from build123d import *

# Parameters (mm, degrees)
ESQUISSE1_W             = 80
ESQUISSE1_H             = 40
BOSS_EXTRU_1_DEPTH      = 2
ESQUISSE2_R             = 1.5
ENL_V_MAT_EXTRU_1_DEPTH = 2
ENL_V_MAT_EXTRU_2_DEPTH = 10


with BuildPart() as part:
    # Esquisse1 → Boss.-Extru.1 (new body)
    with BuildSketch(Plane.XY):
        with Locations((40, 20)):
            Rectangle(ESQUISSE1_W, ESQUISSE1_H)
    extrude(amount=BOSS_EXTRU_1_DEPTH)

    # Esquisse2 → Enlèv. mat.-Extru.1 (cut)
    with BuildSketch(Plane.XY.offset(2)):
        with Locations((2.5, 37.5)):
            Circle(ESQUISSE2_R)
        with Locations((77.5, 37.5)):
            Circle(ESQUISSE2_R)
        with Locations((2.5, 2.5)):
            Circle(ESQUISSE2_R)
        with Locations((77.5, 2.5)):
            Circle(ESQUISSE2_R)
    extrude(amount=-ENL_V_MAT_EXTRU_1_DEPTH, mode=Mode.SUBTRACT)

    # Esquisse3 → Enlèv. mat.-Extru.2 (cut)
    with BuildSketch(Plane(origin=(0, 0, 0), x_dir=(-1, 0, 0), z_dir=(0, 0, -1))):
        Polygon((-25, 40), (-55, 40), (-48.246308582, 33.246308582), (-31.753691418, 33.246308582), align=None)
    extrude(amount=-ENL_V_MAT_EXTRU_2_DEPTH, mode=Mode.SUBTRACT)


solid = part.part
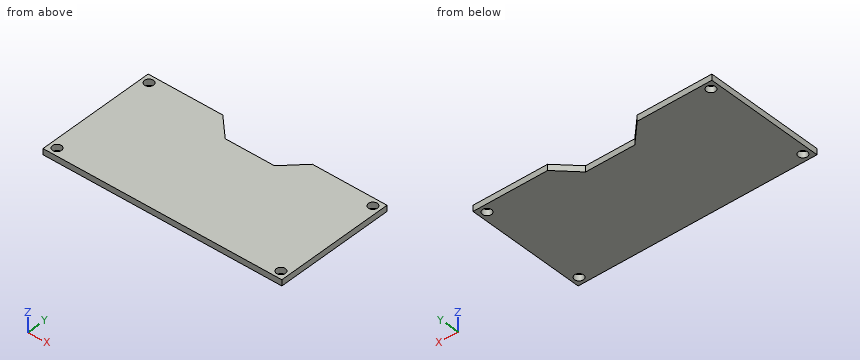
Work out the finished part from the listing and answer in its coordinate system (mm). Give positions to 0.01 mm unless a question says otherwise; leave off trailing zeros. Order: outer loops, then holes, each group sorted by start corner. A loop starts at its lowest first (then second) coordinate and runs counter-clockwise, first axis right, second up. Notation, with made-up numbers: (65, 4.25) -> (120, 4.25) arc R30 ccw to (120, 27.25) -> close; hole circle Ø4 at (26.5, -23.5). An arc over 180 degrees is marked (long way). One line per item, written item: value.
Item 1: Straight lines are drawn through the part: probe 1 along Y at (x, z) = (2.5, 1.1); probe 2 along X at (y, z) = (34, 1.45). For each, find the intervals that lie inside material, in ascending order.
Answer sheet:
probe 1: 0 to 1, 4 to 36, 39 to 40
probe 2: 0 to 31, 49 to 80
Item 2: Find section D-D, the plane z = 1.3. Give the vertices of the cut face in (x, y), plus the area to 3 significant figures.
Answer sheet:
outline: (0, 0) -> (80, 0) -> (80, 40) -> (55, 40) -> (48.25, 33.25) -> (31.75, 33.25) -> (25, 40) -> (0, 40) -> close; hole circle Ø3 at (2.5, 2.5); hole circle Ø3 at (2.5, 37.5); hole circle Ø3 at (77.5, 2.5); hole circle Ø3 at (77.5, 37.5)
area: 3,010 mm²
Item 3: Find section A-A, the plane y = 2.5. Give the vertices of the cut face in (x, z), plus the area to 3 significant figures.
Answer sheet:
outline: (0, 0) -> (1, 0) -> (1, 2) -> (0, 2) -> close; (4, 0) -> (76, 0) -> (76, 2) -> (4, 2) -> close; (79, 0) -> (80, 0) -> (80, 2) -> (79, 2) -> close
area: 148 mm²
Item 4: Find section B-B, the plane y = 37.5. Give the vertices of the cut face in (x, z), plus the area to 3 significant figures.
Answer sheet:
outline: (0, 0) -> (1, 0) -> (1, 2) -> (0, 2) -> close; (4, 0) -> (27.5, 0) -> (27.5, 2) -> (4, 2) -> close; (52.5, 0) -> (76, 0) -> (76, 2) -> (52.5, 2) -> close; (79, 0) -> (80, 0) -> (80, 2) -> (79, 2) -> close
area: 98.0 mm²
Item 5: Find section C-C, the plane x = 77.5. Give the vertices of the cut face in (y, z).
Answer sheet:
outline: (0, 0) -> (1, 0) -> (1, 2) -> (0, 2) -> close; (4, 0) -> (36, 0) -> (36, 2) -> (4, 2) -> close; (39, 0) -> (40, 0) -> (40, 2) -> (39, 2) -> close
